```python
from build123d import *

# Parameters (mm, degrees)
SKETCH1_R           = 1.55
BOSS_EXTRUDE1_DEPTH = 5


with BuildPart() as part:
    # Sketch1 → Boss-Extrude1 (new body)
    with BuildSketch(Plane(origin=(0, 0, 0), x_dir=(1, 0, 0), z_dir=(0, 1, 0))):
        Polygon((-30, 25), (-30, -25), (-20, -25), (-20, -20), (-16.5, -20), (-16.5, -15), (-18, -15), (-18, -12), (-16.5, -12), (-16.5, -8), (-13.5, -8), (-13.5, -12), (-12, -12), (-12, -15), (-13.5, -15), (-13.5, -20), (-10, -20), (-10, -25), (10, -25), (10, -20), (13.5, -20), (13.5, -15), (12, -15), (12, -12), (13.5, -12), (13.5, -8), (16.5, -8), (16.5, -12), (18, -12), (18, -15), (16.5, -15), (16.5, -20), (20, -20), (20, -25), (30, -25), (30, 25), (20, 25), (20, 20), (16.5, 20), (16.5, 15), (18, 15), (18, 12), (16.5, 12), (16.5, 8), (13.5, 8), (13.5, 12), (12, 12), (12, 15), (13.5, 15), (13.5, 20), (10, 20), (10, 25), (-10, 25), (-10, 20), (-13.5, 20), (-13.5, 15), (-12, 15), (-12, 12), (-13.5, 12), (-13.5, 8), (-16.5, 8), (-16.5, 12), (-18, 12), (-18, 15), (-16.5, 15), (-16.5, 20), (-20, 20), (-20, 25), align=None)
        with Locations(Location((4.95, 4.95, 0), (0, 0, 270))):
            Circle(SKETCH1_R, mode=Mode.SUBTRACT)
        with Locations(Location((-4.95, -4.95, 0), (0, 0, 270))):
            Circle(SKETCH1_R, mode=Mode.SUBTRACT)
        with Locations(Location((4.95, -4.95, 0), (0, 0, 270))):
            Circle(SKETCH1_R, mode=Mode.SUBTRACT)
        with Locations(Location((-4.95, 4.95, 0), (0, 0, 270))):
            Circle(SKETCH1_R, mode=Mode.SUBTRACT)
    extrude(amount=BOSS_EXTRUDE1_DEPTH)


solid = part.part
```
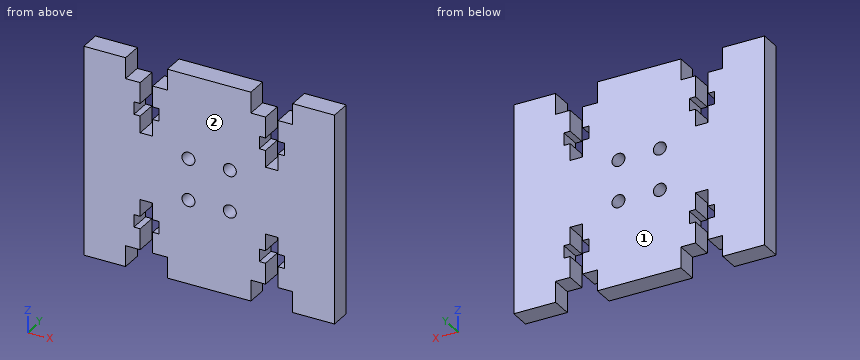
Could you check a few things on this model? Use its own coordinates, in mm. Face numbers are marked on the shaded views. Round coordinates to 2 decimals unless told otherwise and drop trailing zeros. Loops run counter-clockwise (first coordinate to the right, second up) from the corner with the lowest first, then second, coordinate; pieces in that order, holes last.
Q1. Please list where these lines run through material, in increasing order: L1, parallel to X at y = 1.35, z = -4.95; L2, parallel to X at y = 1.25, z = -17.5; L3, parallel to Z at x = 13, y = 3.2.
Q2. I want a section at A-A (z = 4.95). Write out the boundary of the cut face in (x, y), and give its area (3 significant figures).
Q3. I want a section at B-B (x = -4.95). Write out the boundary of the cut face in (y, z).
Q4. I want a section at C-C (y = 4.15). Give the number of separate pieces and of enclosed holes in the cut face, and give its area (3 significant figures).
Q5. For P1, Ø0.8, axis at x = -13, y = 3, coming from the +Z side; P2, Ø2, axis at x = 20, z = 6.5, coming from the -Y side; P3, Ø1.2, axis at x = -13, y = 2.5, coming from the -Z side, each with a flat end and sliding along its axis, tell me the tip position at first contact or that it passes through.
Q6. Thinking about a two-plate mould opening in Y: for the marked faces 1 and 2, which applies, pulls with the +Y half, pulls with the -Y half, needs draft (parallel to the pull), parting line crosses it, or undercut?
Answer below:
1. L1: x = -30 to -6.5, -3.4 to 3.4, 6.5 to 30
1. L2: x = -30 to -16.5, -13.5 to 13.5, 16.5 to 30
1. L3: z = -20 to -15, -12 to 12, 15 to 20
2. outline: (-30, 0) - (-6.5, 0) - (-6.5, 5) - (-30, 5) - close; (-3.4, 0) - (3.4, 0) - (3.4, 5) - (-3.4, 5) - close; (6.5, 0) - (30, 0) - (30, 5) - (6.5, 5) - close
2. area: 269 mm2
3. outline: (0, -25) - (5, -25) - (5, -6.5) - (0, -6.5) - close; (0, -3.4) - (5, -3.4) - (5, 3.4) - (0, 3.4) - close; (0, 6.5) - (5, 6.5) - (5, 25) - (0, 25) - close
4. separate pieces: 1
4. enclosed holes: 4
4. area: 2,590 mm2
5. P1: stops at z = 20
5. P2: stops at y = 0
5. P3: stops at z = -20
6. face 1: pulls with the +Y half
6. face 2: pulls with the -Y half
